For this review, take the finished solid that the model builds, in its own axes (mm). Coordinates: 2 decimals unless noted, no trailing zeros. Loops run counter-clockwise (first coordinate to the right, second up) from the corner with the lowest first, then second, coordinate; pieces in that order, holes last. Notation, with made-up numbers: M 36.25,16 L 66.25,16 A18 cw 66.25,38 Z; hole C 25,72 d4. An arc over 180 degrees is marked long. Answer as a JSON object with one key per item and string values. Group by question number.
Item 1: Wall thickness on L1, parallel to Z at x = 37.5, y = 0; L2, parallel to Z at x = 40, y = 50.5; L3, parallel to Z at x = 31, y = -35: over which ranges is each line inside the solid? List them lowest first. Write a range as from..to.
Item 2: Mouldability with a two-part tool opening along Y and no side actions: class faces 1 (the face through (37.57, -2.75, -12.4)), 2 (the face through (0, -2, -31)), 3 (the face through (37.97, -120.94, -92.73)) as +Y half, -Y half, draft (parallel to the pull), parting line (faces both ways), or undercut.
Item 3: Add section C-C (x = 10.5). State the section outline as (y, z) points, then the cut area to 3 significant figures.
Item 4: Add section A-A (y = 0). State the section outline as (x, z) points.
Item 5: Insertion check: pin 1 (1 mm diameter, centred on x = 19, z = 117.5, fed in from +Y); pin 2 (4 mm diameter, centred on y = -121, z = 87.5, fed in from +X); pin 3 (5 mm diameter, centred on x = 26, z = -105.5, fed in from -Y); pin 4 (15 mm diameter, centred on y = 0, z = 0, fed in from +X). Each pin has a flat end and moves straight along its axis. Give the tip position at first contact, or say it passes through.
from build123d import *

# Parameters (mm, degrees)
F0_R     = 152.4
F0_R_2   = 12.7
F1_DEPTH = 76.2
F2_T     = -2.54
F4_R     = 5.08


# Not quite as in the source:
# - a fillet or chamfer that OpenCascade refuses, or shapes differently, is made with other operations: its cross-section is extruded or revolved along the edge and cut away or added


with BuildPart() as f1:
    # F0 (on Right) → F1 (new body)
    with BuildSketch(Plane.YZ):
        Circle(F0_R)
        Circle(F0_R_2, mode=Mode.SUBTRACT)
    extrude(amount=F1_DEPTH)

    # F2
    f2_openings = [f1.faces().sort_by_distance(p)[0] for p in [
        (76.2, -148.089477, 0),
    ]]
    offset(amount=F2_T, openings=f2_openings)

    # F3: fillet of radius 5.08 on 2 edges, made by hand

    # F3_s1 → F3_t2 (revolve, cut)
    with BuildSketch(Plane.XY):
        with BuildLine():
            ThreePointArc((71.8005909488, 152.4), (74.3405909488, 151.7194090512), (76.2, 149.86))
            Line((76.2, 149.86), (76.2, 152.4))
            Line((76.2, 152.4), (71.8005909488, 152.4))
        make_face()
    revolve(axis=Axis((76.2, 0, 0), (1, 0, 0)), mode=Mode.SUBTRACT)

    # F3_s3 → F3_t4 (revolve, cut)
    with BuildSketch(Plane.XY):
        with BuildLine():
            ThreePointArc((76.2, 12.7), (74.3405909488, 14.5594090512), (71.8005909488, 15.24))
            Line((71.8005909488, 15.24), (76.2, 15.24))
            Line((76.2, 15.24), (76.2, 12.7))
        make_face()
    revolve(axis=Axis((76.2, 0, 0), (1, 0, 0)), mode=Mode.SUBTRACT)

    # F4
    f4_edges = [f1.edges().sort_by_distance(p)[0] for p in [
        (0, -152.4, 0),
        (35.900295, 152.4, 0),
        (71.800591, -152.4, 0),
    ]]
    fillet(f4_edges, radius=F4_R)


solid = f1.part
From the geometry:
{
 "1": {"L1": "z = -152.4..-149.86, -15.24..-12.7, 12.7..15.24, 149.86..152.4", "L2": "z = -143.79..-141.09, 141.09..143.79", "L3": "z = -148.33..-145.72, 145.72..148.33"},
 "2": {"face 1": "undercut", "face 2": "draft", "face 3": "parting line"},
 "3": {"outline": "C 0,0 d304.8; C 0,0 d30.48; hole C 0,0 d299.72; hole C 0,0 d25.4", "area": "2,630 mm²"},
 "4": {"outline": "M 0,-147.32 A5.08 ccw 5.08,-152.4 L 71.8,-152.4 A5.08 ccw 76.2,-149.86 L 2.54,-149.86 L 2.54,-15.24 L 71.8,-15.24 A5.08 ccw 76.2,-12.7 L 0,-12.7 Z; M 0,12.7 L 76.2,12.7 A5.08 ccw 71.8,15.24 L 2.54,15.24 L 2.54,149.86 L 76.2,149.86 A5.08 ccw 71.8,152.4 L 5.08,152.4 A5.08 ccw 0,147.32 Z"},
 "5": {"pin 1": "stops at y = 97.66", "pin 2": "stops at x = 76.2", "pin 3": "stops at y = -112.32", "pin 4": "passes through"}
}
